from build123d import *

# Parameters (mm, degrees)
SKETCH1_W                       = 170
SKETCH1_H                       = 170
BOSS_EXTRUDE1_DEPTH             = 10
F_4_0MM_DOWEL_HOLE1_D           = 4
F_4_0MM_DOWEL_HOLE1_DEPTH       = 5.2
F_4_0MM_DOWEL_HOLE1_TIP         = 1.201721238
CBORE_FOR_M6_SHCS1_D            = 6.6
CBORE_FOR_M6_SHCS1_DEPTH        = 10
CBORE_FOR_M6_SHCS1_CBORE_D      = 11
CBORE_FOR_M6_SHCS1_CBORE_DEPTH  = 6
M3X0_5_TAPPED_HOLE1_D           = 2.5
M3X0_5_TAPPED_HOLE1_DEPTH       = 7.5
M3X0_5_TAPPED_HOLE1_TIP         = 0.751075774
M3X0_5_TAPPED_HOLE2_D           = 2.5
M3X0_5_TAPPED_HOLE2_DEPTH       = 10
M3X0_5_TAPPED_HOLE2_CSINK_D     = 3.05
M3X0_5_TAPPED_HOLE2_CSINK_ANGLE = 90
M3X0_5_TAPPED_HOLE2_TIP         = 0.751075774
M3X0_5_TAPPED_HOLE3_D           = 2.5
M3X0_5_TAPPED_HOLE3_DEPTH       = 10
M3X0_5_TAPPED_HOLE3_CSINK_D     = 3.05
M3X0_5_TAPPED_HOLE3_CSINK_ANGLE = 90
M3X0_5_TAPPED_HOLE3_TIP         = 0.751075774
M3X0_5_TAPPED_HOLE4_D           = 2.5
M3X0_5_TAPPED_HOLE4_DEPTH       = 10
M3X0_5_TAPPED_HOLE4_CSINK_D     = 3.05
M3X0_5_TAPPED_HOLE4_CSINK_ANGLE = 90
M3X0_5_TAPPED_HOLE4_TIP         = 0.751075774
M3X0_5_TAPPED_HOLE5_D           = 2.5
M3X0_5_TAPPED_HOLE5_DEPTH       = 10
M3X0_5_TAPPED_HOLE5_CSINK_D     = 3.05
M3X0_5_TAPPED_HOLE5_CSINK_ANGLE = 90
M3X0_5_TAPPED_HOLE5_TIP         = 0.751075774
M3X0_5_TAPPED_HOLE6_D           = 2.5
M3X0_5_TAPPED_HOLE6_DEPTH       = 8
M3X0_5_TAPPED_HOLE6_CSINK_D     = 3.05
M3X0_5_TAPPED_HOLE6_CSINK_ANGLE = 90
M3X0_5_TAPPED_HOLE6_TIP         = 0.751075774


with BuildPart() as part:
    # Sketch1 → Boss-Extrude1 (new body)
    with BuildSketch(Plane(origin=(0, 0, 0), x_dir=(1, 0, 0), z_dir=(0, 1, 0))):
        with Locations((-21.335769449, -13.148097821)):
            Rectangle(SKETCH1_W, SKETCH1_H)
    extrude(amount=BOSS_EXTRUDE1_DEPTH)

    # Ø4.0mm Dowel Hole1
    with Locations(Plane(origin=(0, 10, 0), x_dir=(1, 0, 0), z_dir=(0, 1, 0))):
        with Locations((2.809433667, -21.75635539), (2.809433667, -39.45635539), (-96.335769449, -18.40635539), (-96.335769449, -43.10635539)):
            Hole(F_4_0MM_DOWEL_HOLE1_D / 2, depth=F_4_0MM_DOWEL_HOLE1_DEPTH)
            with Locations((0, 0, -(F_4_0MM_DOWEL_HOLE1_DEPTH + F_4_0MM_DOWEL_HOLE1_TIP / 2))):  # 118° drill point
                Cone(0, F_4_0MM_DOWEL_HOLE1_D / 2, F_4_0MM_DOWEL_HOLE1_TIP, mode=Mode.SUBTRACT)

    # CBORE for M6 SHCS1
    with Locations(Plane(origin=(0, 0, 0), x_dir=(-1, 0, 0), z_dir=(0, -1, 0))):
        with Locations((96.335769449, -30.75635539), (21.190566333, -39.45635539), (21.190566333, -21.75635539)):
            CounterBoreHole(CBORE_FOR_M6_SHCS1_D / 2, CBORE_FOR_M6_SHCS1_CBORE_D / 2, CBORE_FOR_M6_SHCS1_CBORE_DEPTH, depth=CBORE_FOR_M6_SHCS1_DEPTH)

    # M3x0.5 Tapped Hole1
    with Locations(Plane(origin=(0, 10, 0), x_dir=(1, 0, 0), z_dir=(0, 1, 0))):
        with Locations((-72.324091559, -61.794513309), (-52.324091559, -61.794513309), (-72.324091559, -1.794513309), (-52.324091559, -1.794513309)):
            Hole(M3X0_5_TAPPED_HOLE1_D / 2, depth=M3X0_5_TAPPED_HOLE1_DEPTH)
            with Locations((0, 0, -(M3X0_5_TAPPED_HOLE1_DEPTH + M3X0_5_TAPPED_HOLE1_TIP / 2))):  # 118° drill point
                Cone(0, M3X0_5_TAPPED_HOLE1_D / 2, M3X0_5_TAPPED_HOLE1_TIP, mode=Mode.SUBTRACT)

    # M3x0.5 Tapped Hole2
    with Locations(Plane.XY.offset(98.148097821)):
        with Locations((-96.835769449, 5), (-46.835769449, 5), (4.164230551, 5), (54.164230551, 5)):
            CounterSinkHole(M3X0_5_TAPPED_HOLE2_D / 2, M3X0_5_TAPPED_HOLE2_CSINK_D / 2, depth=M3X0_5_TAPPED_HOLE2_DEPTH, counter_sink_angle=M3X0_5_TAPPED_HOLE2_CSINK_ANGLE)
            with Locations((0, 0, -(M3X0_5_TAPPED_HOLE2_DEPTH + M3X0_5_TAPPED_HOLE2_TIP / 2))):  # 118° drill point
                Cone(0, M3X0_5_TAPPED_HOLE2_D / 2, M3X0_5_TAPPED_HOLE2_TIP, mode=Mode.SUBTRACT)

    # M3x0.5 Tapped Hole3
    with Locations(Plane.ZY.offset(106.335769449)):
        with Locations((-60.851902179, 5), (-10.851902179, 5), (37.148097821, 5), (87.148097821, 5)):
            CounterSinkHole(M3X0_5_TAPPED_HOLE3_D / 2, M3X0_5_TAPPED_HOLE3_CSINK_D / 2, depth=M3X0_5_TAPPED_HOLE3_DEPTH, counter_sink_angle=M3X0_5_TAPPED_HOLE3_CSINK_ANGLE)
            with Locations((0, 0, -(M3X0_5_TAPPED_HOLE3_DEPTH + M3X0_5_TAPPED_HOLE3_TIP / 2))):  # 118° drill point
                Cone(0, M3X0_5_TAPPED_HOLE3_D / 2, M3X0_5_TAPPED_HOLE3_TIP, mode=Mode.SUBTRACT)

    # M3x0.5 Tapped Hole4
    with Locations(Plane(origin=(0, 0, -71.851902179), x_dir=(-1, 0, 0), z_dir=(0, 0, -1))):
        with Locations((-54.164230551, 5), (-4.164230551, 5), (46.835769449, 5), (96.835769449, 5)):
            CounterSinkHole(M3X0_5_TAPPED_HOLE4_D / 2, M3X0_5_TAPPED_HOLE4_CSINK_D / 2, depth=M3X0_5_TAPPED_HOLE4_DEPTH, counter_sink_angle=M3X0_5_TAPPED_HOLE4_CSINK_ANGLE)
            with Locations((0, 0, -(M3X0_5_TAPPED_HOLE4_DEPTH + M3X0_5_TAPPED_HOLE4_TIP / 2))):  # 118° drill point
                Cone(0, M3X0_5_TAPPED_HOLE4_D / 2, M3X0_5_TAPPED_HOLE4_TIP, mode=Mode.SUBTRACT)

    # M3x0.5 Tapped Hole5
    with Locations(Plane(origin=(63.664230551, 0, 0), x_dir=(0, 0, -1), z_dir=(1, 0, 0))):
        with Locations((-83.648097821, 5), (-33.648097821, 5), (7.351902179, 5), (57.351902179, 5)):
            CounterSinkHole(M3X0_5_TAPPED_HOLE5_D / 2, M3X0_5_TAPPED_HOLE5_CSINK_D / 2, depth=M3X0_5_TAPPED_HOLE5_DEPTH, counter_sink_angle=M3X0_5_TAPPED_HOLE5_CSINK_ANGLE)
            with Locations((0, 0, -(M3X0_5_TAPPED_HOLE5_DEPTH + M3X0_5_TAPPED_HOLE5_TIP / 2))):  # 118° drill point
                Cone(0, M3X0_5_TAPPED_HOLE5_D / 2, M3X0_5_TAPPED_HOLE5_TIP, mode=Mode.SUBTRACT)

    # M3x0.5 Tapped Hole6
    with Locations(Plane(origin=(0, 10, 0), x_dir=(1, 0, 0), z_dir=(0, 1, 0))):
        with Locations((34.664230551, 41.851902179), (48.664230551, 16.851902179)):
            CounterSinkHole(M3X0_5_TAPPED_HOLE6_D / 2, M3X0_5_TAPPED_HOLE6_CSINK_D / 2, depth=M3X0_5_TAPPED_HOLE6_DEPTH, counter_sink_angle=M3X0_5_TAPPED_HOLE6_CSINK_ANGLE)
            with Locations((0, 0, -(M3X0_5_TAPPED_HOLE6_DEPTH + M3X0_5_TAPPED_HOLE6_TIP / 2))):  # 118° drill point
                Cone(0, M3X0_5_TAPPED_HOLE6_D / 2, M3X0_5_TAPPED_HOLE6_TIP, mode=Mode.SUBTRACT)


solid = part.part
Part model, mm, in its own coordinate system. A direction names the side the tool comes from. Round coordinates to 2 decimals unless told otherwise and drop trailing zeros. Put each result on its own line as item: value.
Q1. Pull direction Z, two halves, no side cores. Call faces 1 (the face through (-94.338, 7.364, 43.018)), 2 (the face through (63.664, 5, 14)), 3 (the face through (2.76, 3.81, 39.11)), 4 (the face through (-23, 5, -71.852)): pulls with the +Z half, pulls with the -Z half, needs draft (parallel to the pull), parting line crosses it, or undercut.
From the geometry:
face 1: undercut
face 2: needs draft
face 3: undercut
face 4: pulls with the -Z half
Q2. Wall check: line 1 (X direction, y = 5, z = -64.25); line 2 (X direction, y = 6, z = -64); line 3 (Z direction, x = 4.5, y = 8.5) (3 decimals). Give the ranges that are in metal, low to high. Write a range as [from, to].
From the geometry:
line 1: x = [-106.34, -98.09], [-95.59, -48.09], [-45.59, 2.91], [5.41, 52.91], [55.41, 63.66]
line 2: x = [-106.34, -97.59], [-96.09, -47.59], [-46.09, 3.41], [4.91, 53.41], [54.91, 63.66]
line 3: z = [-71.852, 20.688], [22.825, 38.388], [40.525, 98.148]
Q3. Tool access for faces 5 (the face through (-20.5, 3, 34)), 6 (the face through (3.07, 7.364, 37.473)), 7 (the face through (-23, 10, 12)): list every direction of +Z, -Z, +X, -X, +Y, -Y with a clear straight run to the whole face (end or side of a thin tool).
From the geometry:
face 5: -Y
face 6: +Y
face 7: +Z, -Z, +X, -X, +Y
Q4. Pin check, flat tips, straight feed: pin 1 Ø2 at (y, z) = (5, 37.15) entering from -X; pin 2 Ø2 at (x, z) = (34.66, -41.85) entering from +Y; pin 3 Ø2 at (x, y) = (54.16, 5) entering from -Z. Stop position of each tip, or through.
From the geometry:
pin 1: stops at x = -96.19
pin 2: stops at y = 1.85
pin 3: stops at z = -61.7
